Autodesk Fusion 360 part; units mm, degrees
sketch "Sketch2" plane through (0, 0, 0) normal (0, 0, -1) x (1, 0, 0)
  line L0 (0, 0) -> (0, -80)
  line L1 (0, -80) -> (120, -80)
  line L2 (120, -80) -> (120, 0)
  line L3 (120, 0) -> (0, 0)
  line L4 (18, -18.25) -> (108, -18.25)
  line L5 (109.5, -19.75) -> (109.5, -60.25)
  line L6 (108, -61.75) -> (18, -61.75)
  line L7 (16.5, -60.25) -> (16.5, -19.75)
  arc A0 (18, -18.25) -> (16.5, -19.75) centre (18, -19.75) ccw
  arc A1 (16.5, -60.25) -> (18, -61.75) centre (18, -60.25) ccw
  arc A2 (109.5, -19.75) -> (108, -18.25) centre (108, -19.75) ccw
  arc A3 (108, -61.75) -> (109.5, -60.25) centre (108, -60.25) ccw
  point P0 (16.5, -18.25)
  point P1 (109.5, -18.25)
  point P2 (16.5, -61.75)
  dimension "d8" = 93
  dimension "d9" = 43.5
  dimension "d10" = 18.25
  dimension "d11" = 18.25
  dimension "d12" = 16.5
  dimension "d15" = 1.5
  dimension "d16" = 1.5
sketch "Sketch3" plane through (0, 0, 0) normal (0, 0, -1) x (1, 0, 0)
  line L0 (18, -18.25) -> (108, -18.25)
  arc A0 (109.5, -19.75) -> (108, -18.25) centre (108, -19.75) ccw
  line L1 (109.5, -19.75) -> (109.5, -60.25)
  arc A1 (108, -61.75) -> (109.5, -60.25) centre (108, -60.25) ccw
  line L2 (108, -61.75) -> (18, -61.75)
  arc A2 (16.5, -60.25) -> (18, -61.75) centre (18, -60.25) ccw
  line L3 (16.5, -60.25) -> (16.5, -19.75)
  arc A3 (18, -18.25) -> (16.5, -19.75) centre (18, -19.75) ccw
  line L4 (0, 0) -> (0, -80)
  line L5 (0, -80) -> (120, -80)
  line L6 (120, -80) -> (120, 0)
  line L7 (120, 0) -> (0, 0)
  arc A4 (111, -19.75) -> (108, -16.75) centre (108, -19.75) ccw
  line L8 (18, -16.75) -> (108, -16.75)
  arc A5 (18, -16.75) -> (15, -19.75) centre (18, -19.75) ccw
  line L9 (15, -60.25) -> (15, -19.75)
  arc A6 (15, -60.25) -> (18, -63.25) centre (18, -60.25) ccw
  line L10 (108, -63.25) -> (18, -63.25)
  arc A7 (108, -63.25) -> (111, -60.25) centre (108, -60.25) ccw
  line L11 (111, -19.75) -> (111, -60.25)
  dimension "d17" = -1.5
extrude "Extrude3" add sketch "Sketch3" along normal blind 11.5 contours A4 L8 A5 L9 A6 L10 A7 L11
sketch "Sketch4" plane through (0, 16.75, 0) normal (0, -1, 0) x (1, 0, 0)
  line L0 (18, 0) -> (18, -11.5)
  line L1 (18, -11.5) -> (108, -11.5)
  line L2 (108, -11.5) -> (108, 0)
  line L3 (15, 0) -> (15, -1.6) construction
  line L4 (15, -1.6) -> (29.14, -11.5)
  line L5 (15, 0) -> (15, -11.5)
  line L6 (29.14, -11.5) -> (15, -11.5)
  line L7 (15, -1.6) -> (15, -11.5)
  line L8 (108, 0) -> (18, 0)
  point P0 (15, -11.5)
  dimension "d20" = 1.6
  dimension "d21" = 14.14
extrude "Extrude4" cut sketch "Sketch4" against normal up to surface (46.5 mm away) contours L0 L1 L4 L6 | L0 L4 L5 L6 L7
sketch "Sketch5" plane through (0, 0, -11.5) normal (0, 0, -1) x (1, 0, 0)
  line L0 (29.14, -63.25) -> (108, -63.25)
  arc A0 (108, -63.25) -> (111, -60.25) centre (108, -60.25) ccw
  line L1 (111, -60.25) -> (111, -19.75)
  arc A1 (111, -19.75) -> (108, -16.75) centre (108, -19.75) ccw
  line L2 (108, -16.75) -> (29.14, -16.75)
  line L3 (29.14, -18.25) -> (108, -18.25)
  arc A2 (109.5, -19.75) -> (108, -18.25) centre (108, -19.75) ccw
  line L4 (109.5, -19.75) -> (109.5, -60.25)
  arc A3 (108, -61.75) -> (109.5, -60.25) centre (108, -60.25) ccw
  line L5 (108, -61.75) -> (29.14, -61.75)
  line L6 (109.5, -22.75) -> (111, -22.75)
  line L7 (111, -22.75) -> (111, -57.25)
  line L8 (111, -57.25) -> (109.5, -57.25)
  line L9 (109.5, -57.25) -> (109.5, -22.75)
  line L10 (29.14, -16.75) -> (29.14, -18.25)
  line L11 (29.14, -61.75) -> (29.14, -63.25)
  dimension "d26" = 1.5
  dimension "d27" = 34.5
  dimension "d28" = 4.5
  dimension "d29" = 4.5
extrude "Extrude5" add sketch "Sketch5" along normal blind 26.5 contours L1 L4 L6 L7 L8 L9
sketch "Sketch6" plane through (111, 0, 0) normal (1, 0, 0) x (0, 1, 0)
  line L0 (19.75, 0) -> (19.75, -11.5)
  line L1 (19.75, -11.5) -> (22.75, -11.5)
  line L2 (22.75, -11.5) -> (22.75, -38)
  line L3 (22.75, -38) -> (57.25, -38)
  line L4 (57.25, -38) -> (57.25, -11.5)
  line L5 (57.25, -11.5) -> (60.25, -11.5)
  line L6 (60.25, -11.5) -> (60.25, 0)
  line L7 (22.75, -38) -> (57.25, -38)
  line L8 (57.25, -38) -> (57.25, -36.5)
  line L9 (57.25, -36.5) -> (22.75, -36.5)
  line L10 (22.75, -36.5) -> (22.75, -38)
  line L11 (60.25, 0) -> (19.75, 0)
  dimension "d34" = 34.5
  dimension "d35" = 1.5
extrude "Extrude6" add sketch "Sketch6" along normal blind 5 contours L2 L3 L4 L7 L8 L9 L10
fillet "Fillet4" radius 2 2 edges at (116, 57.25, -37.25) (116, 22.75, -37.25)
sketch "Sketch7" plane through (0, 0, 0) normal (0, 0, 1) x (1, 0, 0)
  line L0 (120, 65) -> (10, 65)
  line L1 (10, 65) -> (10, 15)
  line L2 (10, 15) -> (120, 15)
  line L3 (120, 15) -> (120, 65)
extrude "Extrude7" add sketch "Sketch7" along normal blind 1
extrude "Extrude8" cut 1 faces at (78, 32.75, 0) along direction (0, 0, 1) up to surface (1 mm away)
fillet "Fillet5" radius 2 4 edges at (10, 15, 0.5) (120, 15, 0.5) (120, 65, 0.5) (10, 65, 0.5)
equation "d10 = d11"
equation "d28 = d29"
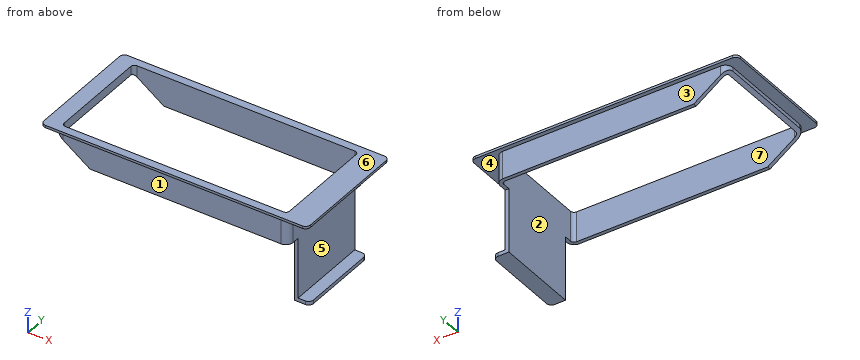
Model file for the job. Use its own axes, mm. Face numbers are marked on the shaded views. A direction names the side the tool comes from. Coordinates: 2 decimals unless noted, no trailing zeros. Order: outer loops, then holes, each group sorted by start corner. A loop starts at its lowest first (then second) coordinate and runs counter-clockwise, first axis right, second up. Notation, with made-up numbers: (-37.5, 66.5) -> (2.5, 66.5) arc R25 ccw to (2.5, 87.5) -> close; hole circle Ø2 at (-33, 28). An arc over 180 degrees is marked (long way). Answer as a JSON object with one key per item and string values. Group by question number.
1) Drill centre lines: L1, parallel to Y at x = 35, z = -6; L2, parallel to X at y = 24.5, z = -16; L3, parallel to X at y = 23, z = -2.5. Where is each one in solid material? Low to high.
2) Flat gauge pins, fed straight in: pin 1 (2 mm diameter, centred on y = 23.5, z = -33.5, fed in from +X); pin 2 (6.5 mm diameter, centred on x = 83, y = 60.5, fed in from -Z); pin 3 (14 mm diameter, centred on x = 59.5, z = -6.5, fed in from -Y); pin 4 (6 mm diameter, centred on x = 45.5, z = -6.5, fed in from +Y). Where does each tip first touch, or does it go through?
3) Cut at C-C, the plane z = -10. Write the cut outline in (x, y).
4) Pull direction Z, two halves, no side cores. Call the marked faces 4, 5, 6 and 7: +Z half, -Z half, draft (parallel to the pull), parting line (faces both ways), or undercut.
5) Which spindle directions (+Z, -Z, +X, -X, +Y, -Y) get a long thin tool onto all of the face, cutting with end or side? Do the marked faces 1, 2 and 3. Say none if no direction does.
6) Cut at B-B, the plane x = 81. Write the cut outline in (y, z), then the cut area to 3 significant figures.
7) Cut at D-D, the plane x = 27. Write the cut outline in (y, z), then the cut area to 3 significant figures.
8) Cut at A-A, the plane y = 30.5. Write the cut outline in (x, z).
Check values:
{
 "1": {"L1": "y = 16.75 to 18.25, 61.75 to 63.25", "L2": "x = 109.5 to 111", "L3": "x = 16.29 to 16.5, 109.5 to 111"},
 "2": {"pin 1": "stops at x = 111", "pin 2": "stops at z = -11.5", "pin 3": "stops at y = 15", "pin 4": "stops at y = 63.25"},
 "3": {"outline": "(27, 16.75) -> (108, 16.75) arc R3 ccw to (111, 19.75) -> (111, 60.25) arc R3 ccw to (108, 63.25) -> (27, 63.25) -> (27, 61.75) -> (108, 61.75) arc R1.5 cw to (109.5, 60.25) -> (109.5, 19.75) arc R1.5 cw to (108, 18.25) -> (27, 18.25) -> close"},
 "4": {"face 4": "undercut", "face 5": "undercut", "face 6": "+Z half", "face 7": "draft"},
 "5": {"face 1": "-Z, +X, -X, -Y", "face 2": "+Z, -Z", "face 3": "-Z, +X, -X, +Y"},
 "6": {"outline": "(15, 0) -> (16.75, 0) -> (16.75, -11.5) -> (18.25, -11.5) -> (18.25, 1) -> (15, 1) -> close; (61.75, -11.5) -> (63.25, -11.5) -> (63.25, 0) -> (65, 0) -> (65, 1) -> (61.75, 1) -> close", "area": "41.0 mm²"},
 "7": {"outline": "(15, 0) -> (16.75, 0) -> (16.75, -10) -> (18.25, -10) -> (18.25, 1) -> (15, 1) -> close; (61.75, -10) -> (63.25, -10) -> (63.25, 0) -> (65, 0) -> (65, 1) -> (61.75, 1) -> close", "area": "36.5 mm²"},
 "8": {"outline": "(10, 0) -> (15, 0) -> (15, -1.6) -> (16.5, -2.65) -> (16.5, 1) -> (10, 1) -> close; (109.5, -38) -> (116, -38) -> (116, -36.5) -> (111, -36.5) -> (111, 0) -> (120, 0) -> (120, 1) -> (109.5, 1) -> close"}
}
